```python
from build123d import *

# Parameters (mm, degrees)
F0_W     = 152.4
F0_H     = 8.58716
F0_W_2   = 187.096558
F0_H_2   = 12.7
F0_W_3   = 127
F0_H_3   = 8.5852
F1_DEPTH = 152.4


with BuildPart() as f1:
    # F0 (on Front) → F1 (new body)
    with BuildSketch(Plane.XZ):
        with Locations((-807.900843, 4.29358)):
            Rectangle(F0_W, F0_H)
        Polygon((-731.700843, 8.58716), (-731.700843, 0), (-69.772355, 0), (-69.772355, 12.7), align=None)
        with Locations((23.775924, 6.35)):
            Rectangle(F0_W_2, F0_H_2)
        Polygon((117.324203, 12.7), (117.324203, 0), (741.499157, 0), (741.499157, 8.5852), align=None)
        with Locations((804.999157, 4.2926)):
            Rectangle(F0_W_3, F0_H_3)
    extrude(amount=F1_DEPTH)


solid = f1.part
```
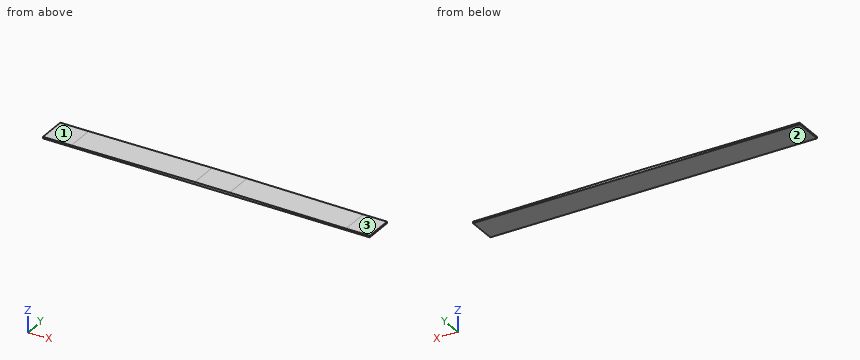
Geometry check sheet. Reference: the model listing, model coordinates, mm. Face numbers are marked on the shaded views. A direction names the side the tool comes from. Round coordinates to 2 decimals unless told otherwise and drop trailing zeros. Loops run counter-clockwise (first coordinate to the right, second up) from the corner with the lowest first, then second, coordinate; pieces in that order, holes last. Notation, with made-up numbers: M 9.5,-28 L 15.5,-28 A30 cw 15.5,11 Z; hole C 74.25,44.5 d6. An arc over 180 degrees is marked long. Return JSON: item names as keys, results as strings. Group by question number.
(1) Section check C-C, the plane x = -689.5. Enter the section's corners in (y, z), and give its area (3 significant figures).
(2) Section check A-A, the plane y = -48. Enter the section's corners in (x, z), and give its area (3 significant figures).
(3) Scan lines: line 1 along Z through (x, y) = (168, -121); line 2 along Z through (x, y) = (642.5, -62). Record each from-to range of solid material in increasing order. Write a range as [from, to].
(4) Set-up check for the marked faces 1, 2 and 3: record each of +Z, -Z, +X, -X, +Y, -Y from which the full face is reachable in a straight line by a thin tool's end or side.
(5) Go/stop test with flat-tipped pins: pin 1 (5 mm diameter, centred on y = -18, z = 10.5, fed in from -X); pin 2 (8 mm diameter, centred on x = -324, y = -52, fed in from +Z); pin 3 (2 mm diameter, centred on x = 407, y = -53, fed in from +Z). Record where each tip stops, or that it passes through.
(6) Section check B-B, the plane x = -501. Enter the section's corners in (y, z), and give its area (3 significant figures).
Data:
{
 "1": {"outline": "M -152.4,0 L 0,0 L 0,8.85 L -152.4,8.85 Z", "area": "1,350 mm²"},
 "2": {"outline": "M -884.1,0 L 868.5,0 L 868.5,8.59 L 741.5,8.59 L 117.32,12.7 L -69.77,12.7 L -731.7,8.59 L -884.1,8.59 Z", "area": "18,500 mm²"},
 "3": {"line 1": "[0, 12.37]", "line 2": "[0, 9.24]"},
 "4": {"face 1": "+Z, -X, +Y, -Y", "face 2": "-Z, +X, -X, +Y, -Y", "face 3": "+Z, +X, +Y, -Y"},
 "5": {"pin 1": "x = -884.1", "pin 2": "z = 11.15", "pin 3": "z = 10.8"},
 "6": {"outline": "M -152.4,0 L 0,0 L 0,10.02 L -152.4,10.02 Z", "area": "1,530 mm²"}
}
